Geometry check sheet. Reference: the model listing, model coordinates, mm. A direction names the side the tool comes from. Coordinates: 2 decimals unless noted, no trailing zeros. Order: outer loops, then holes, each group sorted by start corner. A loop starts at its lowest first (then second) coordinate and runs counter-clockwise, first axis right, second up. Notation, with made-up numbers: (50.25, 8.25) - (64.25, 8.25) arc R18 ccw to (64.25, 40.25) - close; hole circle Ø1 at (3, 77.25). An arc over 180 degrees is marked (long way). Return JSON: item names as keys, results as strings. Group by question number.
Item 1: Tool access check on faces 4 (the flat face through (38, 41, 4.762)), 5 (the flat face through (38, -40, 4.762)), 6 (the flat face through (-39, -38, 4.762)), 7 (the cylindrical face through (-45.84, -48.74, 0.78)). Record the directions out of +Z, -Z, +X, -X, +Y, -Y that give a thin tool (end or side, any length) a straight path to the whole face; none if there is none.
Item 2: Section check A-A on x = -4. Enter the section's corners in (y, z), then the cut area to 3 significant figures.
Item 3: Gauge pin test, flat end, axial feed: pin 1 (4 mm diameter, centred on x = 46.83, y = -46.83, fed in from +Z). Record the tip position at first contact, or that the pin passes through.
Item 4: Section check B-B on z = 3. Enter the section's corners in (x, y).
Item 5: Section check D-D on y = 43. Enter the section's corners in (x, z).
Item 6: Section check C-C on x = 42. Enter the section's corners in (y, z), then the cut area to 3 significant figures.
Item 7: Draft check along X on faces 1 (the cylindrical face through (-11.012, -49.592, 3.153)), 2 (the flat face through (38, -40, 1.588)), 3 (the cylindrical face through (46.36, 44.73, 0.78)). Enter one of: pulls with the +X half, pulls with the -X half, needs draft (parallel to the pull), parting line crosses it, or undercut.
Item 8: Scan lines: probe 1 along Y at (x, z) = (46, 5); probe 2 along Z at (x, y) = (35.5, 40.5); probe 3 along Y at (x, z) = (-13, 5). Record each from-to range of solid material in increasing order.
from build123d import *

# Parameters (mm, degrees)
F0_W     = 101.6
F0_H     = 101.6
F0_R     = 2.15265
F0_R_2   = 38.1
F1_DEPTH = 1.5875
F2_R     = 50.8
F2_R_2   = 38.1
F3_DEPTH = 3.175
F4_W     = 101.6
F4_H     = 101.6
F4_R     = 2.15265
F4_R_2   = 38.1
F5_DEPTH = 1.5875
F6_R     = 3.96875


with BuildPart() as f1:
    # F0 (on Top) → F1 (new body)
    with BuildSketch(Plane.XY):
        Rectangle(F0_W, F0_H)
        with Locations((-46.83125, -46.83125)):
            Circle(F0_R, mode=Mode.SUBTRACT)
        Circle(F0_R_2, mode=Mode.SUBTRACT)
        with Locations((46.83125, -46.83125)):
            Circle(F0_R, mode=Mode.SUBTRACT)
        with Locations((-46.83125, 46.83125)):
            Circle(F0_R, mode=Mode.SUBTRACT)
        with Locations((46.83125, 46.83125)):
            Circle(F0_R, mode=Mode.SUBTRACT)
    extrude(amount=F1_DEPTH)

    # F2 (on face) → F3 (join)
    with BuildSketch(Plane.XY.offset(1.5875)):
        Circle(F2_R)
        Circle(F2_R_2, mode=Mode.SUBTRACT)
    extrude(amount=F3_DEPTH)

    # F4 (on face) → F5 (join)
    with BuildSketch(Plane.XY.offset(4.7625)):
        Rectangle(F4_W, F4_H)
        with Locations((-46.83125, -46.83125)):
            Circle(F4_R, mode=Mode.SUBTRACT)
        Circle(F4_R_2, mode=Mode.SUBTRACT)
        with Locations((46.83125, -46.83125)):
            Circle(F4_R, mode=Mode.SUBTRACT)
        with Locations((-46.83125, 46.83125)):
            Circle(F4_R, mode=Mode.SUBTRACT)
        with Locations((46.83125, 46.83125)):
            Circle(F4_R, mode=Mode.SUBTRACT)
    extrude(amount=F5_DEPTH)

    # F6
    f6_edges = [f1.edges().sort_by_distance(p)[0] for p in [
        (-50.8, 50.8, 0.79375),
        (-50.8, -50.8, 0.79375),
        (50.8, -50.8, 0.79375),
        (50.8, 50.8, 0.79375),
        (-50.8, 50.8, 5.55625),
        (-50.8, -50.8, 5.55625),
        (50.8, -50.8, 5.55625),
        (50.8, 50.8, 5.55625),
    ]]
    fillet(f6_edges, radius=F6_R)


solid = f1.part
Computed:
{
 "1": {"face 4": "+X, +Y", "face 5": "+X, -Y", "face 6": "-X, -Y", "face 7": "+Z, -Z"},
 "2": {"outline": "(-50.8, 0) - (-37.89, 0) - (-37.89, 6.35) - (-50.8, 6.35) - (-50.8, 4.76) - (-50.64, 4.76) - (-50.64, 1.59) - (-50.8, 1.59) - close; (37.89, 0) - (50.8, 0) - (50.8, 1.59) - (50.64, 1.59) - (50.64, 4.76) - (50.8, 4.76) - (50.8, 6.35) - (37.89, 6.35) - close", "area": "163 mm²"},
 "3": {"pin 1": "passes through"},
 "4": {"outline": "circle Ø101.6 at (0, 0); hole circle Ø76.2 at (0, 0)"},
 "5": {"outline": "(-50.8, 0) - (50.8, 0) - (50.8, 1.59) - (27.05, 1.59) - (27.05, 4.76) - (50.8, 4.76) - (50.8, 6.35) - (-50.8, 6.35) - (-50.8, 4.76) - (-27.05, 4.76) - (-27.05, 1.59) - (-50.8, 1.59) - close"},
 "6": {"outline": "(-50.8, 0) - (50.8, 0) - (50.8, 1.59) - (28.58, 1.59) - (28.58, 4.76) - (50.8, 4.76) - (50.8, 6.35) - (-50.8, 6.35) - (-50.8, 4.76) - (-28.58, 4.76) - (-28.58, 1.59) - (-50.8, 1.59) - close", "area": "504 mm²"},
 "7": {"face 1": "parting line crosses it", "face 2": "needs draft", "face 3": "undercut"},
 "8": {"probe 1": "y = -50.8 to -48.82, -44.85 to 44.85, 48.82 to 50.8", "probe 2": "z = 0 to 1.59, 4.76 to 6.35", "probe 3": "y = -50.8 to -35.81, 35.81 to 50.8"}
}
